Can you work these out from the drawing? Everything is in mm from the part's minimum corner. A direction names the side the tool comes from. Give positions to 0.01 mm unless a question says otherwise; leave off trailing zeros. Order: outer loops, then holes, each group sorted by start corner. A loop starts at its lowest first (then second) coordinate and runs counter-clockwise, first axis right, second up. Notation, with made-up numbers: M 56.5,22.5 L 60.5,22.5 A35 cw 60.5,57.5 Z; hole C 32.25,58 d6. An arc over 180 degrees is marked long. Answer as a JSON object with one key per item and string values.
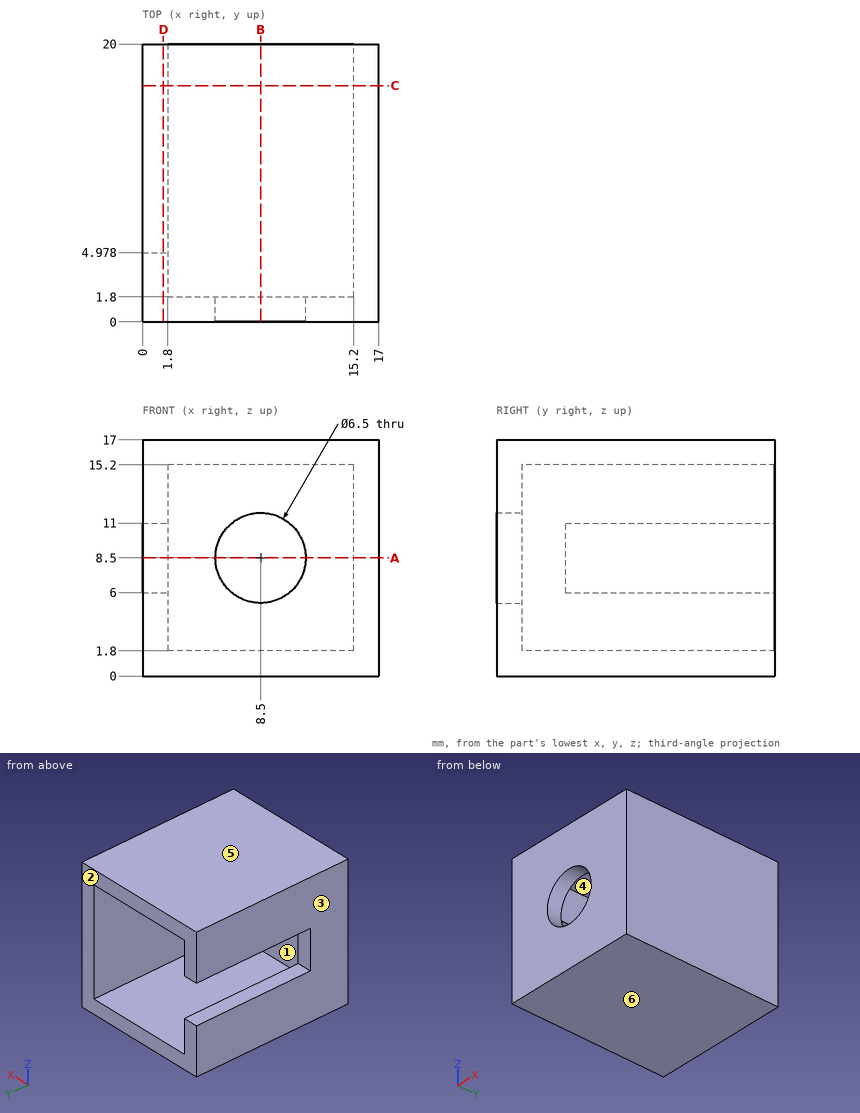
1) I'm going to push flat-ended pins straight in: pin 1 Ø4 at (x, z) = (6, 10) entering from +Y; pin 2 Ø6.5 at (x, y) = (5.5, 9.5) entering from -Z; pin 3 Ø0.9 at (x, z) = (1, 9) entering from +Y. Where does each tip first touch, or does it pass through?
Results found:
{"pin 1": "stops at y = 1.8", "pin 2": "stops at z = 0", "pin 3": "stops at y = 4.98"}
2) For the marked faces 1 and 2, which set-ups out of +Z, -Z, +X, -X, +Y, -Y let a thin tool reach every point of the face, with its end or its side?
Results found:
{"face 1": "+Y", "face 2": "+Z, -Z, +X, -X, +Y"}
3) I want a section at A-A on z = 8.5. Write out the boundary of the cut face in (x, y).
Results found:
{"outline": "M 0,0 L 5.25,0 L 5.25,1.8 L 1.8,1.8 L 1.8,4.98 L 0,4.98 Z; M 11.75,0 L 17,0 L 17,20 L 15.2,20 L 15.2,1.8 L 11.75,1.8 Z"}
4) Thinking about a two-plate mould opening in Z: for the marked faces 3, 4, 5 and 6, which applies, pulls with the +Z half, pulls with the -Z half, needs draft (parallel to the pull), parting line crosses it, or undercut?
Results found:
{"face 3": "needs draft", "face 4": "undercut", "face 5": "pulls with the +Z half", "face 6": "pulls with the -Z half"}
5) I want a section at C-C on y = 17. Write out the boundary of the cut face in (x, z).
Results found:
{"outline": "M 0,0 L 17,0 L 17,17 L 0,17 L 0,11 L 1.8,11 L 1.8,15.2 L 15.2,15.2 L 15.2,1.8 L 1.8,1.8 L 1.8,6 L 0,6 Z"}
6) I want a section at D-D on x = 1.5. Write out the boundary of the cut face in (y, z), and give its area (3 significant figures).
Results found:
{"outline": "M 0,0 L 20,0 L 20,6 L 4.98,6 L 4.98,11 L 20,11 L 20,17 L 0,17 Z", "area": "265 mm²"}
7) I want a section at B-B on x = 8.5. Write out the boundary of the cut face in (y, z).
Results found:
{"outline": "M 0,0 L 20,0 L 20,1.8 L 1.8,1.8 L 1.8,5.25 L 0,5.25 Z; M 0,11.75 L 1.8,11.75 L 1.8,15.2 L 20,15.2 L 20,17 L 0,17 Z"}
8) I need wall thicknesses on L1, parallel to Z at x = 8.5, y = 0.5; L2, parallel to X at y = 12, z = 4. Which ranges of each line are inside material? Lowest first, please.
Results found:
{"L1": "z = 0 to 5.25, 11.75 to 17", "L2": "x = 0 to 1.8, 15.2 to 17"}
